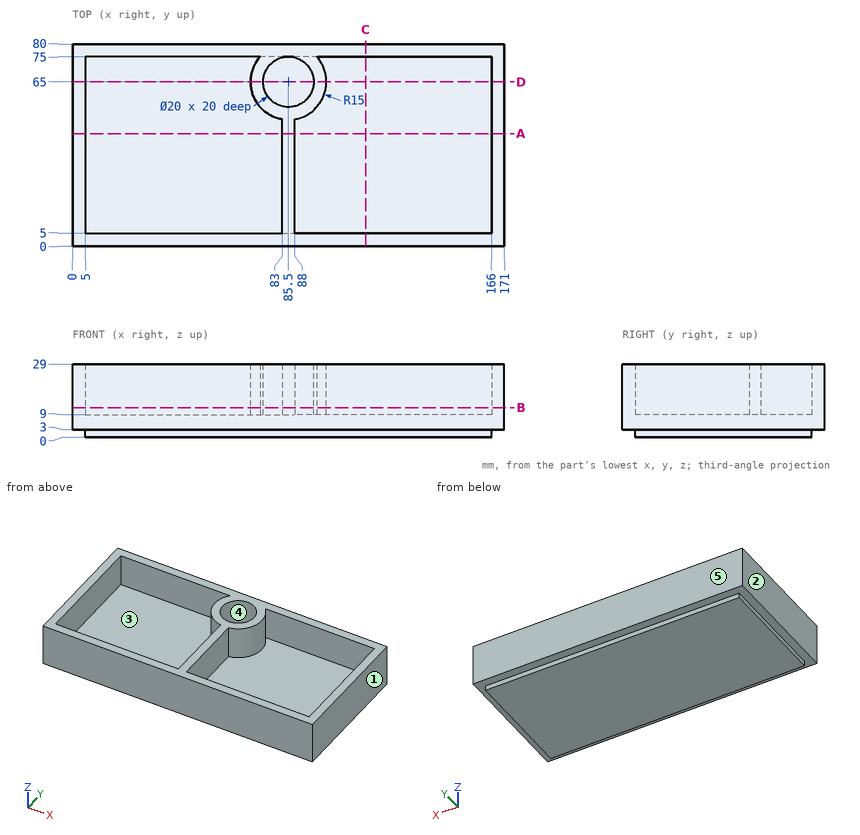
Geometry: see drawing. Coordinates: mm, zero at the bounding-box minimum. A direction names the side the tool comes from. Give positions to 0.01 mm unless a question says otherwise; leave off trailing zeros. Order: outer loops, then holes, each group sorted by start corner. A loop starts at its lowest first (then second) coordinate and runs counter-clockwise, first axis right, second up.
Q1. Contact query for flat-ended pins moving along their axis: pin 1 Ø0.9 at (x, z) = (98.5, 1.5) entering from -Y; pin 2 Ø16 at (x, z) = (33, 18.5) entering from -Y; pin 3 Ø0.9 at (y, z) = (49.5, 1.5) entering from -X; pin 4 Ø6 at (x, y) = (88, 62) entering from +Z. Output: stop coordinate, or through.
Checked values:
pin 1: stops at y = 5
pin 2: stops at y = 0
pin 3: stops at x = 5
pin 4: stops at z = 9
Q2. Ray query, probe 1 along X at (y, z) = (65, 14); probe 2 along X at (y, z) = (17, 22.25); probe 3 along Y at (x, z) = (85.5, 15.5). Return the intervals inside material, ascending.
Checked values:
probe 1: x = 0 to 5, 70.5 to 75.5, 95.5 to 100.5, 166 to 171
probe 2: x = 0 to 5, 83 to 88, 166 to 171
probe 3: y = 0 to 55, 75 to 80
Q3. Draft query along X for the marked faces 1, 2 and 3. Return one class per face: +X half, -X half, draft (parallel to the pull), parting line (faces both ways), or undercut.
Checked values:
face 1: +X half
face 2: -X half
face 3: undercut
Q4. Section C-C on x = 116. Output: boundary loops of the cut face in (y, z), and give its area (3 significant figures).
Checked values:
outline: (0, 3) - (5, 3) - (5, 0) - (75, 0) - (75, 3) - (80, 3) - (80, 29) - (75, 29) - (75, 9) - (5, 9) - (5, 29) - (0, 29) - close
area: 890 mm2
Q5. Section D-D on y = 65. Output: boundary loops of the cut face in (x, z), and give its area (3 significant figures).
Checked values:
outline: (0, 3) - (5, 3) - (5, 0) - (166, 0) - (166, 3) - (171, 3) - (171, 29) - (166, 29) - (166, 9) - (100.5, 9) - (100.5, 29) - (95.5, 29) - (95.5, 9) - (75.5, 9) - (75.5, 29) - (70.5, 29) - (70.5, 9) - (5, 9) - (5, 29) - (0, 29) - close
area: 1,910 mm2
Q6. Section A-A on y = 44.5. Output: boundary loops of the cut face in (x, z), and give its area (3 significant figures).
Checked values:
outline: (0, 3) - (5, 3) - (5, 0) - (166, 0) - (166, 3) - (171, 3) - (171, 29) - (166, 29) - (166, 9) - (88, 9) - (88, 29) - (83, 29) - (83, 9) - (5, 9) - (5, 29) - (0, 29) - close
area: 1,810 mm2
Q7. Section B-B on z = 11.75. Output: boundary loops of the cut face in (x, y).
Checked values:
outline: (0, 0) - (171, 0) - (171, 80) - (0, 80) - close; hole (5, 5) - (83, 5) - (83, 50.21) arc R15 cw to (74.32, 75) - (5, 75) - close; hole circle Ø20 at (85.5, 65); hole (88, 5) - (166, 5) - (166, 75) - (96.68, 75) arc R15 cw to (88, 50.21) - close
Q8. Set-up query: the marked faces 4 and 5. Return all of +Z, -Z, +X, -X, +Y, -Y with unobstructed straight access to the full face (end or side cutting, diameter ignored); none if empty.
Checked values:
face 4: +Z
face 5: +Z, -Z, +X, -X, +Y
